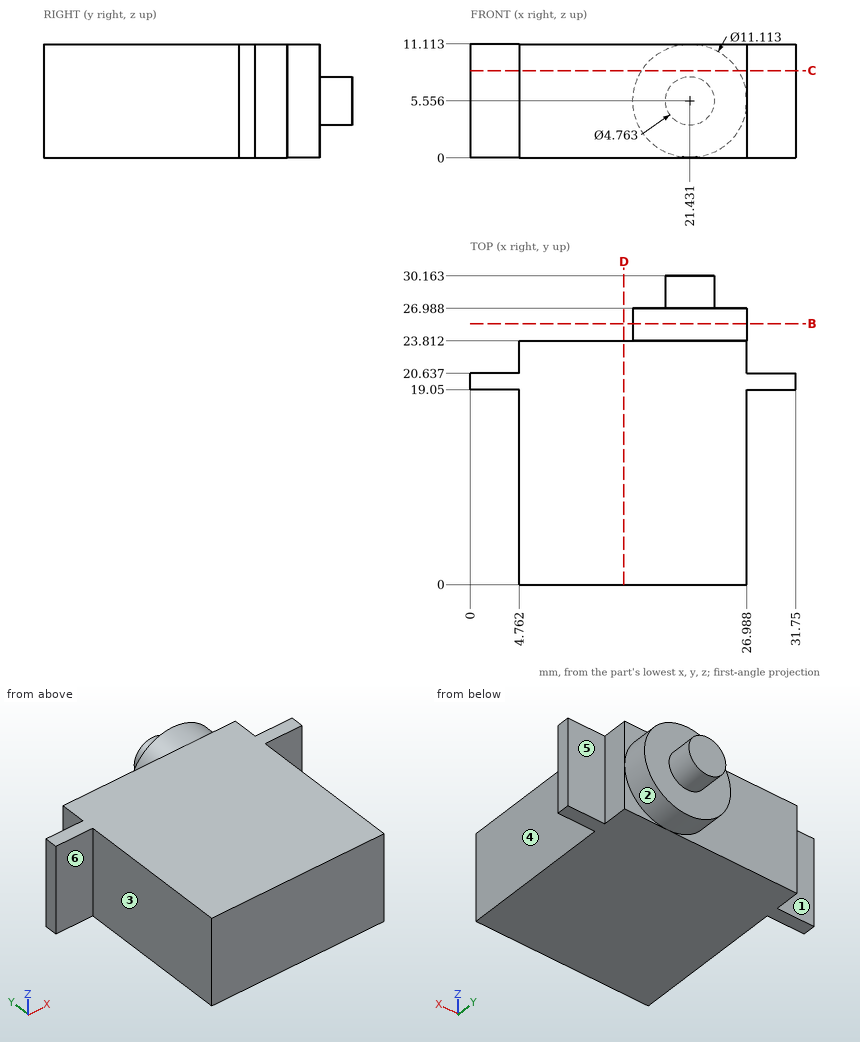
The drawing under review shows one solid part. Ordinate dimensions are in mm from its lowest x, y, z. A direction names the side the tool comes from. Coordinates: 2 decimals unless noted, no trailing zeros. Write each loop counter-clockwise with the first axis right and the second up, starting at its lowest first coordinate (ties: lowest second). Pieces come first, ordered by that corner, then holes. Notation, with made-up numbers: (16.5, 15.25) - (22.5, 15.25) arc R6 ccw to (22.5, 25.25) - close; hole circle Ø6 at (-26.75, -6). An arc over 180 degrees is marked (long way). Answer in a Markdown table with one row per item. Add a question column.
Q1. We need section C-C, the plane z = 8.5. State the section outline as (x, y) points, and give its area (3 significant figures).
Q2. Draft analysis for pull direction Y (two halves, no side actions). For the marked faces 4, 5 and 6, state which applies: +Y half, -Y half, draft (parallel to the pull), parting line (faces both ways), or undercut.
Q3. We need section B-B, the plane y = 25.5. State the section outline as (x, z) points.
Q4. For P1, Ø2.5, axis at x = 2.5, z = 8, coming from the -Y side; P2, Ø3, axis at x = 11, z = 5.5, coming from the -Y side; P3, Ø2.5, axis at y = 22, z = 5.5, coming from the -X side; P4, Ø3.5, axis at y = 6.5, z = 5, coming from the +X side, all flat-tipped, find the tip position at first contact; note any pin that passes through.
Q5. For probe 1 along Y at (x, z) = (11, 8.5); probe 2 along X at (y, z) = (13, 8.75); probe 3 along Y at (x, z) = (21.5, 2), list the stretches that pass through material, from the lowest coordinate up.
Q6. We need section D-D, the plane x = 15. State the section outline as (y, z) points.
Q7. Tool access review of the marked faces 1, 2 and 3: name each direction out of +Z, -Z, +X, -X, +Y, -Y from which nothing blocks a thin tool from reaching the whole face with its end or side.
Answer list:
| question | item | result |
|---|---|---|
| 1 | outline | (0, 19.05) - (4.76, 19.05) - (4.76, 0) - (26.99, 0) - (26.99, 19.05) - (31.75, 19.05) - (31.75, 20.64) - (26.99, 20.64) - (26.99, 23.81) - (26.14, 23.81) - (26.14, 26.99) - (16.72, 26.99) - (16.72, 23.81) - (4.76, 23.81) - (4.76, 20.64) - (0, 20.64) - close |
| 1 | area | 574 mm2 |
| 2 | face 4 | draft |
| 2 | face 5 | +Y half |
| 2 | face 6 | -Y half |
| 3 | outline | circle Ø11.11 at (21.43, 5.56) |
| 4 | P1 | stops at y = 19.05 |
| 4 | P2 | stops at y = 0 |
| 4 | P3 | stops at x = 4.76 |
| 4 | P4 | stops at x = 26.99 |
| 5 | probe 1 | y = 0 to 23.81 |
| 5 | probe 2 | x = 4.76 to 26.99 |
| 5 | probe 3 | y = 0 to 26.99 |
| 6 | outline | (0, 0) - (23.81, 0) - (23.81, 11.11) - (0, 11.11) - close |
| 7 | face 1 | +Z, -Z, -X, +Y |
| 7 | face 2 | +Y |
| 7 | face 3 | +Z, -Z, -X, -Y |
